For this review, take the finished solid that the model builds, in its own axes (mm). A direction names the side the tool comes from. Give positions to 0.01 mm unless a question says otherwise; leave off trailing zeros. Write each loop counter-clockwise with the first axis right and the second up, starting at its lowest first coordinate (ties: lowest second). Pieces come first, ordered by that corner, then holes.
Q1. We need section A-A (x = 17). Write out the cut boundary in (y, z).
Q2. We need section D-D (x = 38). Write out the cut boundary in (y, z), then the cut area to 3 significant figures.
Q3. We need section B-B (z = -3.5). Write out the cut boundary in (x, y), then the cut area to 3 significant figures.
Q4. Machinability: for faces 1 (the flat face through (-32, 6, 35)), 2 (the cylindrical face through (-32.278, 5.451, 24.505)), 3 (the flat face through (-29.82, 3.97, -28.26)), 4 (the flat face through (-32, 7, 38.116)), which of the approach directions +Z, -Z, +X, -X, +Y, -Y give a long, thin tool a straight path to every point of the face, cutting with its end or side? Answer none if there is none.
Q5. We need section C-C (z = 32). Give the number of separate pieces and of enclosed holes in the cut face, then the cut area to 3 significant figures.
Q6. Mouldability with a two-part tool opening along X and no side actions: class faces 5 (the flat face through (-33, 6, -34)), 6 (the flat face through (-32.1, 9, 29.7)) as released by +X, released by -X, zero draft, split by the parting line, or undercut.
Q7. For line 1 (X direction, y = 1, z = -32); line 2 (Z direction, x = -32, y = 8.25), list the stretches that pass through material, from the lowest coordinate up.
Q8. Insertion check: P1, Ø2, axis at x = -31, y = 7.5, coming from the -Z side; P2, Ø3, axis at y = 5, z = -37, coming from the +X side; P3, Ø1.5, axis at x = 34, y = 7.5, coming from the +Z side. Each pin has a flat end and moves straight along its axis. Give the tip position at first contact, or say it passes through.
Autodesk Inventor part; units mm, degrees
ref_plane "YZ Plane" through (0, 0, 0) normal (1, 0, 0) x (0, 1, 0)
ref_plane "XZ Plane" through (0, 0, 0) normal (0, 1, 0) x (-1, 0, 0)
ref_plane "XY Plane" through (0, 0, 0) normal (0, 0, 1) x (1, 0, 0)
sketch "Esquisse1" plane through (0, 0, 0) normal (0, 1, 0) x (-1, 0, 0)
  line L0 (50, 50) -> (-50, 50)
  line L1 (-50, 50) -> (-50, -50)
  line L2 (-50, -50) -> (50, -50)
  line L3 (50, -50) -> (50, 50)
  point P0 (0, 0)
  dimension "d0" = 100
  dimension "d1" = 100
  dimension "d17" = 50
  dimension "d18" = 50
extrude "Extrusion1" add sketch "Esquisse1" along normal blind 2
sketch "Esquisse2" plane through (0, 2, 0) normal (0, 1, 0) x (1, 0, 0)
  line L0 (50, -50) -> (50, 50)
  line L1 (-50, -50) -> (50, -50)
  arc A0 (36.32, -38.1309) -> (27.6597, -38.1165) centre (32, -32) ccw
  line L2 (27.68, -29.4825) -> (32.0203, -27)
  line L3 (32.0203, -27) -> (36.3403, -29.5175)
  line L4 (36.3403, -29.5175) -> (36.32, -34.5175)
  line L5 (27.6597, -34.4825) -> (27.68, -29.4825)
  line L6 (27.6597, -34.4825) -> (27.6597, -38.1165)
  line L7 (36.32, -34.5175) -> (36.32, -38.1309)
  line L8 (53.6963, 0) -> (-74.6388, 0)
  line L9 (0, -61.7794) -> (0, 59.6738)
  arc A1 (-27.6597, -38.1165) -> (-36.32, -38.1309) centre (-32, -32) ccw
  line L10 (-27.68, -29.4825) -> (-32.0203, -27)
  line L11 (-32.0203, -27) -> (-36.3403, -29.5175)
  line L12 (-36.3403, -29.5175) -> (-36.32, -34.5175)
  line L13 (-27.6597, -34.4825) -> (-27.68, -29.4825)
  line L14 (-27.6597, -34.4825) -> (-27.6597, -38.1165)
  line L15 (-36.32, -34.5175) -> (-36.32, -38.1309)
  arc A2 (27.6597, 38.1165) -> (36.32, 38.1309) centre (32, 32) ccw
  line L16 (27.68, 29.4825) -> (32.0203, 27)
  line L17 (32.0203, 27) -> (36.3403, 29.5175)
  line L18 (36.3403, 29.5175) -> (36.32, 34.5175)
  line L19 (27.6597, 34.4825) -> (27.68, 29.4825)
  line L20 (27.6597, 34.4825) -> (27.6597, 38.1165)
  line L21 (36.32, 34.5175) -> (36.32, 38.1309)
  arc A3 (-36.32, 38.1309) -> (-27.6597, 38.1165) centre (-32, 32) ccw
  line L22 (-27.68, 29.4825) -> (-32.0203, 27)
  line L23 (-32.0203, 27) -> (-36.3403, 29.5175)
  line L24 (-36.3403, 29.5175) -> (-36.32, 34.5175)
  line L25 (-27.6597, 34.4825) -> (-27.68, 29.4825)
  line L26 (-27.6597, 34.4825) -> (-27.6597, 38.1165)
  line L27 (-36.32, 34.5175) -> (-36.32, 38.1309)
  point P0 (0, 0)
  dimension "d6" = 18
  dimension "d7" = 18
  dimension "d8" = 15
  dimension "d9" = 5
extrude "Extrusion2" add sketch "Esquisse2" along normal blind 4 contours L7 L4 L3 L2 L5 L6 A0 | L14 L13 L10 L11 L12 L15 A1 | L20 L19 L16 L17 L18 L21 A2 | L27 L24 L23 L22 L25 L26 A3
sketch "Esquisse4" plane through (0, 6, 0) normal (0, 1, 0) x (1, 0, 0)
  arc A0 (36.32, -38.1309) -> (27.6597, -38.1165) centre (32, -32) ccw
  line L0 (27.6597, -38.1165) -> (36.3403, -38.1165)
  line L1 (53.7761, 0) -> (-84.9694, 0)
  line L2 (0, -51.9111) -> (0, 71.3221)
  arc A1 (-27.6597, -38.1165) -> (-36.32, -38.1309) centre (-32, -32) ccw
  line L3 (-27.6597, -38.1165) -> (-36.3403, -38.1165)
  arc A2 (27.6597, 38.1165) -> (36.32, 38.1309) centre (32, 32) ccw
  line L4 (27.6597, 38.1165) -> (36.3403, 38.1165)
  arc A3 (-36.32, 38.1309) -> (-27.6597, 38.1165) centre (-32, 32) ccw
  line L5 (-27.6597, 38.1165) -> (-36.3403, 38.1165)
  point P0 (0, 0)
extrude "Extrusion3" add sketch "Esquisse4" along normal blind 3
sketch "Esquisse5" plane through (0, 9, 0) normal (0, 1, 0) x (1, 0, 0)
  circle A0 centre (32, -32) radius 2
  arc A1 (36.3403, -38.1165) -> (27.6597, -38.1165) centre (32, -32) ccw
  line L0 (0, -51.4977) -> (0, 66.0278)
  line L1 (54.9768, 0) -> (-89.9714, 0)
  circle A2 centre (-32, -32) radius 2
  arc A3 (-27.6597, -38.1165) -> (-36.3403, -38.1165) centre (-32, -32) ccw
  circle A4 centre (32, 32) radius 2
  arc A5 (27.6597, 38.1165) -> (36.3403, 38.1165) centre (32, 32) ccw
  circle A6 centre (-32, 32) radius 2
  arc A7 (-36.3403, 38.1165) -> (-27.6597, 38.1165) centre (-32, 32) ccw
  point P0 (0, 0)
  dimension "d14" = 4
extrude "Extrusion4" cut sketch "Esquisse5" against normal through all
properties part number "support-balise"
Computed:
1. outline: (0, -50) - (2, -50) - (2, 50) - (0, 50) - close
2. outline: (0, -50) - (2, -50) - (2, -36.5) - (9, -36.5) - (9, -27.5) - (2, -27.5) - (2, 27.5) - (9, 27.5) - (9, 36.5) - (2, 36.5) - (2, 50) - (0, 50) - close
2. area: 326 mm2
3. outline: (-50, 0) - (50, 0) - (50, 2) - (-50, 2) - close
3. area: 200 mm2
4. face 1: +Z
4. face 2: +Y
4. face 3: -Z
4. face 4: +Z, +X, -X, +Y
5. separate pieces: 3
5. enclosed holes: 0
5. area: 301 mm2
6. face 5: undercut
6. face 6: zero draft
7. line 1: x = -50 to -34, -30 to 30, 34 to 50
7. line 2: z = -38.12 to -34, -30 to -24.5, 24.5 to 30, 34 to 38.12
8. P1: stops at z = -38.12
8. P2: stops at x = 38.63
8. P3: stops at z = 38.12
